```python
from build123d import *

# Parameters (mm, degrees)
R_VOLUTION1_ANGLE            = 270
ENL_V_MAT_EXTRU_1_DEPTH      = 158.508729917
ENL_V_MAT_EXTRU_1_DEPTH_BACK = 158.508729917
CONG_1_R                     = 2
ESQUISSE6_R                  = 3.75
ENL_V_MAT_EXTRU_2_DEPTH      = 139.115893365
R_P_TITION_CIRCULAIRE2_COUNT = 12
ENL_V_MAT_EXTRU_3_DEPTH      = 131.613532807
ENL_V_MAT_EXTRU_3_DEPTH_BACK = 131.613532807
ESQUISSE9_R                  = 30
ENL_V_MAT_EXTRU_4_DEPTH      = 158.508730061
ENL_V_MAT_EXTRU_4_DEPTH_BACK = 10
CONG_2_R                     = 1


with BuildPart() as part:
    # Esquisse1 → Révolution1 (revolve)
    with BuildSketch(Plane.XY):
        Polygon((0, 0), (-117.728055077, 0), (-117.728055077, 25), (-96.728055077, 25), (-96.728055077, 40), (-65.228055077, 40), (-62.728055077, 37.5), (-25.728055077, 37.5), (-23.228055077, 40), (8.271944923, 40), (8.271944923, 25), (29.271944923, 25), (29.271944923, 0), align=None)
    revolve(axis=Axis((0, 0, 0), (-1, 0, 0)), revolution_arc=R_VOLUTION1_ANGLE)

    # Esquisse3 → Enlèv. mat.-Extru.1 (cut, two sides: drawn at the far end of the back side and taken through both)
    with BuildSketch(Plane.ZY.offset(117.728055077).offset(-ENL_V_MAT_EXTRU_1_DEPTH_BACK)):
        with BuildLine():
            Line((-12, 13), (0, 13))
            ThreePointArc((0, 13), (3, 10), (0, 7))
            Line((0, 7), (-12, 7))
            ThreePointArc((-12, 7), (-15, 10), (-12, 13))
        make_face()
    extrude(amount=ENL_V_MAT_EXTRU_1_DEPTH + ENL_V_MAT_EXTRU_1_DEPTH_BACK, mode=Mode.SUBTRACT)

    # Congé1
    cong_1_edges = [part.edges().sort_by_distance(p)[0] for p in [
        (8.271944923, -17.67766953, -17.67766953),
        (-96.728055077, -17.67766953, -17.67766953),
    ]]
    fillet(cong_1_edges, radius=CONG_1_R)

    # Esquisse6 → Enlèv. mat.-Extru.2 (cut, symmetric)
    with BuildSketch(Plane.ZY.offset(96.728055077)):
        with Locations((-8.282209443, 30.909626441)):
            Circle(ESQUISSE6_R)
    enl_v_mat_extru_2 = extrude(amount=ENL_V_MAT_EXTRU_2_DEPTH, both=True, mode=Mode.SUBTRACT)

    # Répétition circulaire2: Enlèv. mat.-Extru.2 ×12 about axis
    r_p_tition_circulaire2_axis = Axis((0, 0, 0), (1, 0, 0))
    for i in range(1, R_P_TITION_CIRCULAIRE2_COUNT):
        add(enl_v_mat_extru_2.rotate(r_p_tition_circulaire2_axis, i * 360 / R_P_TITION_CIRCULAIRE2_COUNT), mode=Mode.SUBTRACT)

    # Esquisse9 → Enlèv. mat.-Extru.3 (cut, two sides: drawn at the far end of the back side and taken through both)
    with BuildSketch(Plane(origin=(0, 0, 0), x_dir=(1, 0, 0), z_dir=(0, 1, 0)).offset(-ENL_V_MAT_EXTRU_3_DEPTH_BACK)):
        with Locations((29.271944923, -40)):
            Circle(ESQUISSE9_R)
        with BuildLine():
            Line((29.271944923, -40), (23.194258704, -5.531728645))
            ThreePointArc((23.194258704, -5.531728645), (7.965294907, -12.23263309), (-2.448827624, -25.208360839))
            Line((-2.448827624, -25.208360839), (29.271944923, -40))
        make_face()
        with BuildLine():
            Line((29.271944923, -10), (29.271944923, -25))
            Line((29.271944923, -25), (29.271944923, -40))
            Line((29.271944923, -40), (8.271944923, -40))
            Line((8.271944923, -40), (-0.728055077, -40))
            ThreePointArc((-0.728055077, -40), (29.271944923, -70), (59.271944923, -40))
            ThreePointArc((59.271944923, -40), (50.485148358, -18.786796564), (29.271944923, -10))
        make_face()
        with BuildLine():
            Line((-0.728055077, -40), (8.271944923, -40))
            Line((8.271944923, -40), (8.271944923, -30.207539179))
            Line((8.271944923, -30.207539179), (2.082711311, -27.321452148))
            ThreePointArc((2.082711311, -27.321452148), (-0.016935291, -33.506811582), (-0.728055077, -40))
        make_face()
        with BuildLine():
            Line((26.627040212, -25), (29.271944923, -25))
            Line((29.271944923, -25), (29.271944923, -10))
            ThreePointArc((29.271944923, -10), (26.65727264, -10.114159057), (24.062499593, -10.45576741))
            Line((24.062499593, -10.45576741), (26.627040212, -25))
        make_face()
        with BuildLine():
            Line((10.271944923, -25), (26.627040212, -25))
            Line((26.627040212, -25), (24.062499593, -10.45576741))
            ThreePointArc((24.062499593, -10.45576741), (11.009102052, -16.199399791), (2.082711311, -27.321452148))
            Line((2.082711311, -27.321452148), (8.271944923, -30.207539179))
            Line((8.271944923, -30.207539179), (8.271944923, -27))
            ThreePointArc((8.271944923, -27), (8.85773136, -25.585786438), (10.271944923, -25))
        make_face()
    extrude(amount=ENL_V_MAT_EXTRU_3_DEPTH + ENL_V_MAT_EXTRU_3_DEPTH_BACK, mode=Mode.SUBTRACT)

    # Esquisse10 → Enlèv. mat.-Extru.4 (cut, two sides: drawn at the far end of the back side and taken through both)
    with BuildSketch(Plane.ZY.offset(117.728055077).offset(-ENL_V_MAT_EXTRU_4_DEPTH_BACK)):
        with BuildLine():
            Line((-4.776313653, 3), (-19.908574626, 3))
            ThreePointArc((-19.908574626, 3), (-3.674077438, -18.363865829), (18.989837064, -4))
            Line((18.989837064, -4), (-4.776313653, -4))
            Line((-4.776313653, -4), (-4.776313653, 3))
        make_face()
    extrude(amount=ENL_V_MAT_EXTRU_4_DEPTH + ENL_V_MAT_EXTRU_4_DEPTH_BACK, mode=Mode.SUBTRACT)

    # Congé2
    cong_2_edges = [part.edges().sort_by_distance(p)[0] for p in [
        (-107.728055077, 3, -12.342444139),
        (-107.728055077, -18.363865829, -3.674077438),
        (-107.728055077, -0.5, -4.776313653),
        (-107.728055077, -4, 7.106761705),
    ]]
    fillet(cong_2_edges, radius=CONG_2_R)


solid = part.part
```
Build history of the part. All positions in model axes, mm. A direction names the side the tool comes from. Coordinates: 2 decimals unless noted, no trailing zeros. Order: outer loops, then holes, each group sorted by start corner. A loop starts at its lowest first (then second) coordinate and runs counter-clockwise, first axis right, second up. Notation, with made-up numbers: (26, -7.5) -> (61, -7.5) arc R23 ccw to (61, 25.5) -> close; hole circle Ø1 at (-31.75, 41.25). An arc over 180 degrees is marked (long way). Answer in a Markdown table with one row per item. Add a question column.
Q1. Band-saw the part on A-A, the plane x = 18. List the corners of the cut face in (y, z), then the cut area to 3 significant figures.
Q2. Band-saw the part on B-B, the plane x = -49. Give the number of separate pieces and of enclosed holes in the cut face, then the cut area to 3 significant figures.
Q3. Which spindle directions (+Z, -Z, +X, -X, +Y, -Y) get a long thin tool onto all of the face, cutting with end or side? Do faces 1 (the face through (-44, -25.6, -27.4)), 2 (the face through (-43, 4, 0)), 3 (the face through (-43, 13, -6)). Say none if no direction does.
Q4. Mould opens along Z. For faces 4 (the face through (-45, -34.5, -7.2)), 5 (the face through (-108.095, -17.085, -18.251)), 6 (the face through (-96.728, -18, -21)) say: +Z half, -Z half, draft (parallel to the pull), parting line (faces both ways), or undercut.
Q5. Wall check: line 1 along Z through (x, y) = (-61.5, -8); line 2 along Y through (x, z) = (-5, -28); line 3 along Z through (x, y) = (-6.5, -7.5). Give the ranges that are in metal, low to high. Write a range as [from, to].
Q6. Drop flat-ended pins along their axis: pin 1 (12 mm diameter, centred on y = -8.28, z = -30.91, fed in from -X); pin 2 (1 mm diameter, centred on x = -81, z = -9.5, fed in from -Y); pin 3 (9.5 mm diameter, centred on x = -67, z = -6.5, fed in from +Y). Give the stop position or say it passes through.
Answers follow:
| question | item | result |
|---|---|---|
| 1 | outline | (-24.04, 6.86) arc R25 ccw (long way) to (25, 0) -> (13, 0) -> (13, -12) arc R3 cw to (7, -12) -> (7, 0) -> (0, 0) -> (0, 6.86) -> close |
| 1 | area | 1,070 mm^2 |
| 2 | separate pieces | 1 |
| 2 | enclosed holes | 9 |
| 2 | area | 2,830 mm^2 |
| 3 | face 1 | none |
| 3 | face 2 | +Z, +X, -X, +Y |
| 3 | face 3 | +Z, +X, -X |
| 4 | face 4 | undercut |
| 4 | face 5 | parting line |
| 4 | face 6 | draft |
| 5 | line 1 | [-36.64, -34.65], [-27.17, 27.17], [34.65, 36.64] |
| 5 | line 2 | [-28.57, -10.65], [-5.92, 5.92], [10.65, 28.57] |
| 5 | line 3 | [-39.29, -34.58], [-27.24, 27.24], [34.58, 39.29] |
| 6 | pin 1 | x = -97 |
| 6 | pin 2 | y = -38.97 |
| 6 | pin 3 | y = 39.96 |
